Geometry: final body of the model. Coordinates: model frame, mm. Face numbers are marked on the shaded views. Coordinates: 2 decimals unless noted, no trailing zeros. Order: outer loops, then holes, each group sorted by start corner. A loop starts at its lowest first (then second) coordinate and runs counter-clockwise, first axis right, second up. Notation, with made-up numbers: (15.5, 9) -> (61.5, 9) arc R17 ccw to (61.5, 35) -> close; hole circle Ø5 at (87, -16.75). An arc over 180 degrees is marked (long way). Answer in a Markdown table with one row per item. Add a question column.
1) Section query C-C on z = -0.45. Return the cut outline in (x, y), then the cut area to 3 significant figures.
2) Section query D-D on x = -19. Count the separate pieces of the cut face and the enclosed holes in it, then the cut area to 3 significant figures.
3) Ray query, line 1 (Y direction, x = 0, z = -1.5); line 2 (X direction, y = -20, z = 0.65); line 3 (Y direction, x = -17, z = 0.1). Return the intervals inside material, ascending. Write a range as from..to.
4) Pull-direction query (X, two-part tool) for the marked faces 1 and 2; classes: +X half, -X half, draft (parallel to the pull), parting line (faces both ways), or undercut.
5) Section query A-A on y = -20. Return the cut outline in (x, z).
6) Contact query for flat-ended pins moving along their axis: P1, Ø7, axis at x = -20, y = 20, coming from the +Z side; P2, Ø8, axis at x = -20, y = -20, coming from the +Z side. Output: stop coordinate, or through.
7) Section query B-B on x = 0. Return the cut outline in (y, z).
```python
from build123d import *

# Parameters (mm, degrees)
SKETCH1_W           = 60
SKETCH1_H           = 60
BOSS_EXTRUDE1_DEPTH = 1.708
SKETCH2_R           = 3
CUT_EXTRUDE1_DEPTH  = 4.416
CHAMFER1_SIZE       = 3


with BuildPart() as part:
    # Sketch1 → Boss-Extrude1 (new body, symmetric)
    with BuildSketch(Plane.XY):
        Rectangle(SKETCH1_W, SKETCH1_H)
    extrude(amount=BOSS_EXTRUDE1_DEPTH, both=True)

    # Sketch2 → Cut-Extrude1 (cut, through all)
    with BuildSketch(Plane.XY.offset(1.708)):
        with Locations((0, 20)):
            Circle(SKETCH2_R)
        with Locations((0, -20)):
            Circle(SKETCH2_R)
        with Locations((20, -20)):
            Circle(SKETCH2_R)
        with Locations((-20, -20)):
            Circle(SKETCH2_R)
        with Locations((-20, 20)):
            Circle(SKETCH2_R)
        with Locations((20, 20)):
            Circle(SKETCH2_R)
    extrude(amount=-CUT_EXTRUDE1_DEPTH, mode=Mode.SUBTRACT)

    # Chamfer1
    chamfer1_edges = [part.edges().sort_by_distance(p)[0] for p in [
        (-3, -20, 1.708),
        (17, -20, 1.708),
        (-23, -20, 1.708),
        (-23, 20, 1.708),
        (17, 20, 1.708),
        (-3, 20, 1.708),
    ]]
    chamfer(chamfer1_edges, length=CHAMFER1_SIZE)


solid = part.part
```
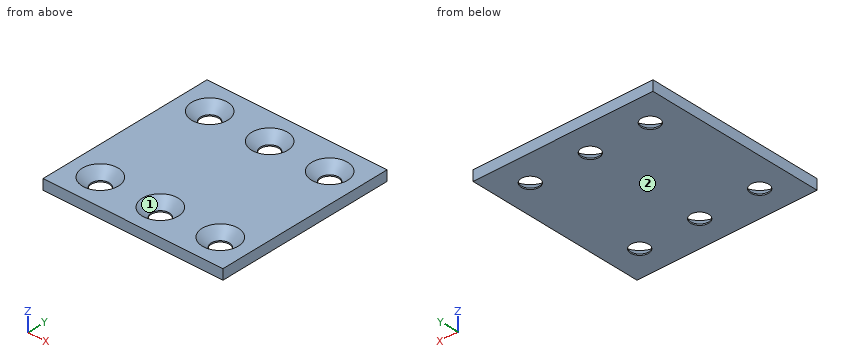
Result:
| question | item | result |
|---|---|---|
| 1 | outline | (-30, -30) -> (30, -30) -> (30, 30) -> (-30, 30) -> close; hole circle Ø7.68 at (-20, -20); hole circle Ø7.68 at (-20, 20); hole circle Ø7.68 at (0, -20); hole circle Ø7.68 at (0, 20); hole circle Ø7.68 at (20, -20); hole circle Ø7.68 at (20, 20) |
| 1 | area | 3,320 mm2 |
| 2 | separate pieces | 3 |
| 2 | enclosed holes | 0 |
| 2 | area | 148 mm2 |
| 3 | line 1 | -30..-23, -17..17, 23..30 |
| 3 | line 2 | -30..-24.94, -15.06..-4.94, 4.94..15.06, 24.94..30 |
| 3 | line 3 | -30..-23.21, -16.79..16.79, 23.21..30 |
| 4 | face 1 | undercut |
| 4 | face 2 | draft |
| 5 | outline | (-30, -1.71) -> (-23, -1.71) -> (-23, -1.29) -> (-26, 1.71) -> (-30, 1.71) -> close; (-17, -1.71) -> (-3, -1.71) -> (-3, -1.29) -> (-6, 1.71) -> (-14, 1.71) -> (-17, -1.29) -> close; (3, -1.71) -> (17, -1.71) -> (17, -1.29) -> (14, 1.71) -> (6, 1.71) -> (3, -1.29) -> close; (23, -1.71) -> (30, -1.71) -> (30, 1.71) -> (26, 1.71) -> (23, -1.29) -> close |
| 6 | P1 | z = -0.79 |
| 6 | P2 | z = -0.29 |
| 7 | outline | (-30, -1.71) -> (-23, -1.71) -> (-23, -1.29) -> (-26, 1.71) -> (-30, 1.71) -> close; (-17, -1.71) -> (17, -1.71) -> (17, -1.29) -> (14, 1.71) -> (-14, 1.71) -> (-17, -1.29) -> close; (23, -1.71) -> (30, -1.71) -> (30, 1.71) -> (26, 1.71) -> (23, -1.29) -> close |
